Source: three-view drawing plus pictorial views. Frame: mm from the lowest corner of the part. Give positions to 0.01 mm unless a question says otherwise; leave off trailing zeros. Loops run counter-clockwise (first coordinate to the right, second up) from the corner with the lowest first, then second, coordinate; pieces in that order, holes last.
1. Material intervals for line 1 along X through (y, z) = (1.4, 1.6); line 2 along X through (y, z) = (1.1, 2.1), sorted ascending.
2. Section B-B, the plane z = 0.35. Output: boundary loops of the cut face in (x, y), then the cut area to 3 significant figures.
3. Section A-A, the plane y = 0.6. Output: boundary loops of the cut face in (x, z).
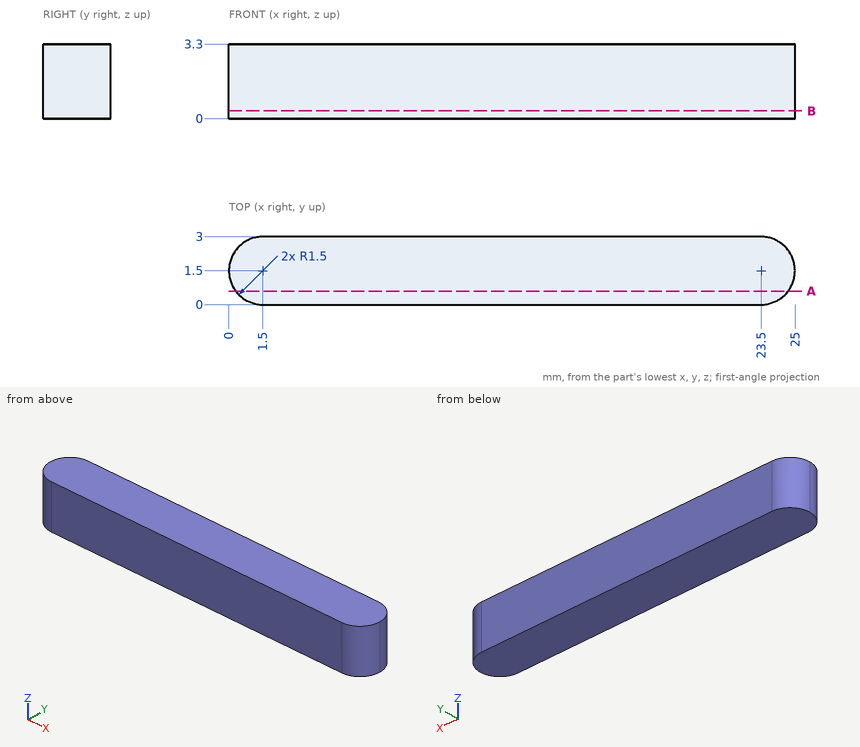
Answers below:
1. line 1: x = 0 to 25
1. line 2: x = 0.05 to 24.95
2. outline: (0, 1.5) arc R1.5 ccw to (1.5, 0) - (23.5, 0) arc R1.5 ccw to (25, 1.5) arc R1.5 ccw to (23.5, 3) - (1.5, 3) arc R1.5 ccw to start
2. area: 73.1 mm2
3. outline: (0.3, 0) - (24.7, 0) - (24.7, 3.3) - (0.3, 3.3) - close
